from build123d import *

# Parameters (mm, degrees)
F0_R     = 13
F0_R_2   = 11.5
F1_DEPTH = 4
F0_R_3   = 6
F0_R_4   = 4.265
F0_R_5   = 11.25
F0_R_6   = 6.25
F2_DEPTH = 3.5


with BuildPart() as f1:
    # F0 (on Top) → F1 (new body, symmetric)
    with BuildSketch(Plane.XY):
        Circle(F0_R)
        Circle(F0_R_2, mode=Mode.SUBTRACT)
    extrude(amount=F1_DEPTH, both=True)



with BuildPart() as f1b:
    # F0 (on Top) → F1, piece 2 (new body, symmetric)
    with BuildSketch(Plane.XY):
        Circle(F0_R_3)
        Circle(F0_R_4, mode=Mode.SUBTRACT)
    extrude(amount=F1_DEPTH, both=True)


with BuildPart() as f1c:
    # F0 (on Top) → F1, piece 3 (new body, symmetric)
    with BuildSketch(Plane.XY):
        Circle(F0_R_5)
        Circle(F0_R_6, mode=Mode.SUBTRACT)
    extrude(amount=F1_DEPTH, both=True)


with BuildPart() as f1_1:
    add(f1.part)

    add(f1b.part)  # F2 merges F1b

    add(f1c.part)  # F2 merges F1c
    # F0 (on Top) → F2 (join, symmetric)
    with BuildSketch(Plane.XY):
        Circle(F0_R_2)
        Circle(F0_R_5, mode=Mode.SUBTRACT)
        Circle(F0_R_6)
        Circle(F0_R_3, mode=Mode.SUBTRACT)
    extrude(amount=F2_DEPTH, both=True)


solid = f1_1.part
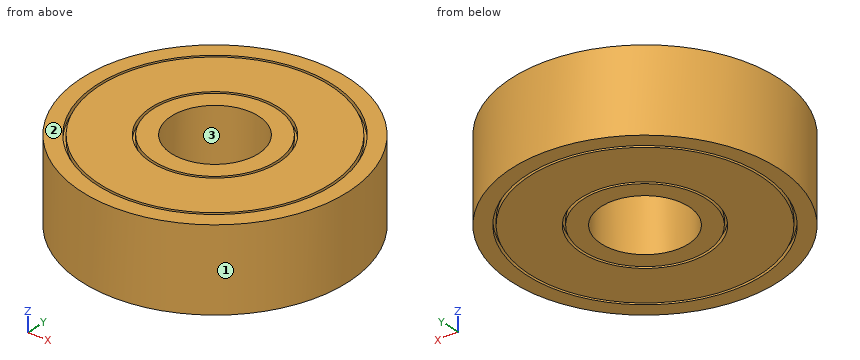
Can you work these out from the model? Positions are in its coordinate system, mm. Face numbers are marked on the shaded views. Coordinates: 2 decimals unless noted, no trailing zeros. Order: outer loops, then holes, each group sorted by start corner. A loop starts at its lowest first (then second) coordinate and runs counter-clockwise, first axis right, second up. Notation, with made-up numbers: M -38.75,-1 L -5.75,-1 A17 cw -5.75,3 Z; hole C 2.5,-33.75 d5. An arc over 180 degrees is marked long. Write item = value, one per line.
(1) Suppose I cut it at B-B on y = 8. Please give me the cut outline in (x, z), plus the area to 3 significant figures.
Results are:
outline = M -10.25,-4 L -8.26,-4 L -8.26,-3.5 L -7.91,-3.5 L -7.91,-4 L 7.91,-4 L 7.91,-3.5 L 8.26,-3.5 L 8.26,-4 L 10.25,-4 L 10.25,4 L 8.26,4 L 8.26,3.5 L 7.91,3.5 L 7.91,4 L -7.91,4 L -7.91,3.5 L -8.26,3.5 L -8.26,4 L -10.25,4 Z
area = 163 mm2
(2) For pin 1 Ø1.5 at (y, z) = (2, 2) entering from +X; pin 2 Ø11 at (x, y) = (0, 0) entering from -Z; pin 3 Ø1.5 at (x, z) = (-6, 3) entering from +Y; pin 4 Ø1 at (y, z) = (2.5, -2) entering from +X, each with a flat end and sliding along its axis, tell me the tip position at first contact or that it passes through.
Results are:
pin_1 = 12.94
pin_2 = -4
pin_3 = 11.89
pin_4 = 12.85
(3) I need wall thicknesses on line 1 along Y through (x, z) = (0, -3.75) (3 decimals); line 2 along Y through (x, z) = (0, -1.75) (3 decimals); line 3 along X through (y, z) = (-10, 3.75). Which ranges of each line are inside material? Lowest first, please. Write a range as [from, to].
Results are:
line_1 = [-13, -11.5], [-11.25, -6.25], [-6, -4.265], [4.265, 6], [6.25, 11.25], [11.5, 13]
line_2 = [-13, -4.265], [4.265, 13]
line_3 = [-8.31, -5.68], [-5.15, 5.15], [5.68, 8.31]
(4) Suppose I cut it at A-A on z = -1.75. Please give me the cut outline in (x, y) (3 decimals), plus the area to 3 significant figures.
Results are:
outline = C 0,0 d26; hole C 0,0 d8.53
area = 474 mm2
(5) Suppose I cut it at C-C on x = 7.5. Please give me the cut outline in (y, z), plus the area to 3 significant figures.
Results are:
outline = M -10.62,-4 L -8.72,-4 L -8.72,-3.5 L -8.39,-3.5 L -8.39,-4 L 8.39,-4 L 8.39,-3.5 L 8.72,-3.5 L 8.72,-4 L 10.62,-4 L 10.62,4 L 8.72,4 L 8.72,3.5 L 8.39,3.5 L 8.39,4 L -8.39,4 L -8.39,3.5 L -8.72,3.5 L -8.72,4 L -10.62,4 Z
area = 169 mm2
(6) If we mould it in two halves opening along Y, with no side actions, what happens to the marked faces 1, 2 and 3? For each: pulls with the +Y half, pulls with the -Y half, needs draft (parallel to the pull), parting line crosses it, or undercut.
Results are:
face_1 = parting line crosses it
face_2 = needs draft
face_3 = undercut
